Here's how the part is built. I have some questions about the finished solid (model axes, mm). A direction names the side the tool comes from. Round coordinates to 2 decimals unless told otherwise and drop trailing zeros. Order: outer loops, then holes, each group sorted by start corner. A loop starts at its lowest first (then second) coordinate and runs counter-clockwise, first axis right, second up. Notation, with made-up numbers: M 29.5,67 L 74.5,67 A14 cw 74.5,76 Z; hole C 9,78 d7. An arc over 180 degrees is marked long. Write item = value, one per line. Start each with the question number.
Item 1: I'm going to push flat-ended pins straight in: P1, Ø1.6, axis at x = 33, y = 6.5, coming from the +Z side; P2, Ø1.3, axis at x = -33, y = -6.5, coming from the +Z side; P3, Ø0.6, axis at x = 33, y = -6.5, coming from the +Z side. Where does each tip first touch, or does it pass through?
Item 2: I want a section at A-A, the plane y = 0. List the corners of the cut face in (x, z) for me.
Item 3: We'd pull the mould along Y, two halves only. Please class faces 1 (the face through (-30, 0, 7)), 2 (the face through (33, 6.5, 6)), 3 (the face through (0, 8.5, 4)): pulls with the +Y half, pulls with the -Y half, needs draft (parallel to the pull), parting line crosses it, or undercut.
Item 4: Please list where these lines run through material, in increasing order: L1, parallel to X at y = 0, z = 4.4; L2, parallel to Y at x = -33, z = 7.8; L3, parallel to Y at x = -14, z = 2.35.
Item 5: I want a section at C-C, the plane y = 3. List the corners of the cut face in (x, z) for me, plus the area to 3 significant figures.
Item 6: I want a section at D-D, the plane x = -21. List the corners of the cut face in (y, z) for me.
Item 7: I want a section at B-B, the plane x = -33. List the corners of the cut face in (y, z) for me, plus the area to 3 significant figures.
Item 8: For faces 4 (the face through (0, 0, 6)), 5 (the face through (-32.446, -6.73, 7.318)), 6 (the face through (35, 0, 4)), which set-ups out of +Z, -Z, +X, -X, +Y, -Y let a thin tool reach every point of the face, with its end or its side?
```python
from build123d import *

# Parameters (mm, degrees)
SKETCH_W        = 70
SKETCH_H        = 17
PAD_DEPTH       = 6
SKETCH001_W     = 5
SKETCH001_H     = 17
PAD001_DEPTH    = 3
SKETCH002_R     = 0.6
POCKET_DEPTH    = 4
SKETCH003_R     = 1.35
POCKET001_DEPTH = 9.001
CHAMFER_SIZE    = 0.4


with BuildPart() as part:
    # Sketch (on XY_Plane of Origin) → Pad (new body)
    with BuildSketch(Plane.XY):
        Rectangle(SKETCH_W, SKETCH_H)
    extrude(amount=PAD_DEPTH)

    # Sketch001 (on Face6 of Pad) → Pad001 (join)
    with BuildSketch(Plane.XY.offset(6)):
        with Locations((-32.5, 0)):
            Rectangle(SKETCH001_W, SKETCH001_H)
    extrude(amount=PAD001_DEPTH)

    # Sketch002 (on Face5 of Pad001) → Pocket (cut)
    with BuildSketch(Plane.XY.offset(9)):
        with Locations((-33, 6.5)):
            Circle(SKETCH002_R)
        with Locations((-33, -6.5)):
            Circle(SKETCH002_R)
    extrude(amount=-POCKET_DEPTH, mode=Mode.SUBTRACT)

    # Mirrored: part across YZ


with BuildPart() as part_1:
    add(part.part)
    add(part.part.mirror(Plane.YZ))

    # Sketch003 (on Face1 of Mirrored) → Pocket001 (cut, through all)
    with BuildSketch(Plane(origin=(0, 0, 0), x_dir=(1, 0, 0), z_dir=(0, 0, -1))):
        with Locations((-14, 0)):
            Circle(SKETCH003_R)
        with Locations((3.5, 0)):
            Circle(SKETCH003_R)
    extrude(amount=-POCKET001_DEPTH, mode=Mode.SUBTRACT)

    # Chamfer
    chamfer_edges = [part_1.edges().sort_by_distance(p)[0] for p in [
        (0, -8.5, 6),
        (-30, -8.5, 7.5),
        (-32.5, -8.5, 9),
        (-30, 0, 9),
        (-30, 0, 6),
        (-35, -8.5, 4.5),
        (0, -8.5, 0),
        (-35, 0, 9),
        (-32.5, 8.5, 9),
        (0, 8.5, 6),
        (-30, 8.5, 7.5),
        (32.5, -8.5, 9),
        (30, 0, 9),
        (30, -8.5, 7.5),
        (35, -8.5, 4.5),
        (35, 0, 9),
        (35, 0, 0),
        (35, 8.5, 4.5),
        (32.5, 8.5, 9),
        (33.6, 6.5, 9),
        (33.6, -6.5, 9),
        (-33.6, 6.5, 9),
        (-33.6, -6.5, 9),
        (-35, 8.5, 4.5),
        (0, 8.5, 0),
        (-35, 0, 0),
        (-15.35, 0, 0),
        (2.15, 0, 0),
    ]]
    chamfer(chamfer_edges, length=CHAMFER_SIZE)


solid = part_1.part
```
Filled in:
q1.P1 = 8.8
q1.P2 = 8.65
q1.P3 = 6
q2.outline = M -35,0.4 L -34.6,0 L -15.75,0 L -15.35,0.4 L -15.35,6 L -29.6,6 L -30,6.4 L -30,8.6 L -30.4,9 L -34.6,9 L -35,8.6 Z; M -12.65,0.4 L -12.25,0 L 1.75,0 L 2.15,0.4 L 2.15,6 L -12.65,6 Z; M 4.85,0.4 L 5.25,0 L 34.6,0 L 35,0.4 L 35,8.6 L 34.6,9 L 30.4,9 L 30,8.6 L 30,6 L 4.85,6 Z
q3.face_1 = needs draft
q3.face_2 = undercut
q3.face_3 = pulls with the +Y half
q4.L1 = -35 to -15.35, -12.65 to 2.15, 4.85 to 35
q4.L2 = -8.5 to -7.1, -5.9 to 5.9, 7.1 to 8.5
q4.L3 = -8.5 to -1.35, 1.35 to 8.5
q5.outline = M -35,0.4 L -34.6,0 L 34.6,0 L 35,0.4 L 35,8.6 L 34.6,9 L 30.4,9 L 30,8.6 L 30,6 L -29.6,6 L -30,6.4 L -30,8.6 L -30.4,9 L -34.6,9 L -35,8.6 Z
q5.area = 450 mm^2
q6.outline = M -8.5,0.4 L -8.1,0 L 8.1,0 L 8.5,0.4 L 8.5,5.6 L 8.1,6 L -8.1,6 L -8.5,5.6 Z
q7.outline = M -8.5,0.4 L -8.1,0 L 8.1,0 L 8.5,0.4 L 8.5,8.6 L 8.1,9 L 7.5,9 L 7.1,8.6 L 7.1,6 L 5.9,6 L 5.9,8.6 L 5.5,9 L -5.5,9 L -5.9,8.6 L -5.9,6 L -7.1,6 L -7.1,8.6 L -7.5,9 L -8.1,9 L -8.5,8.6 Z
q7.area = 145 mm^2
q8.face_4 = +Z, +Y, -Y
q8.face_5 = +Z
q8.face_6 = +Z, -Z, +X, +Y, -Y
